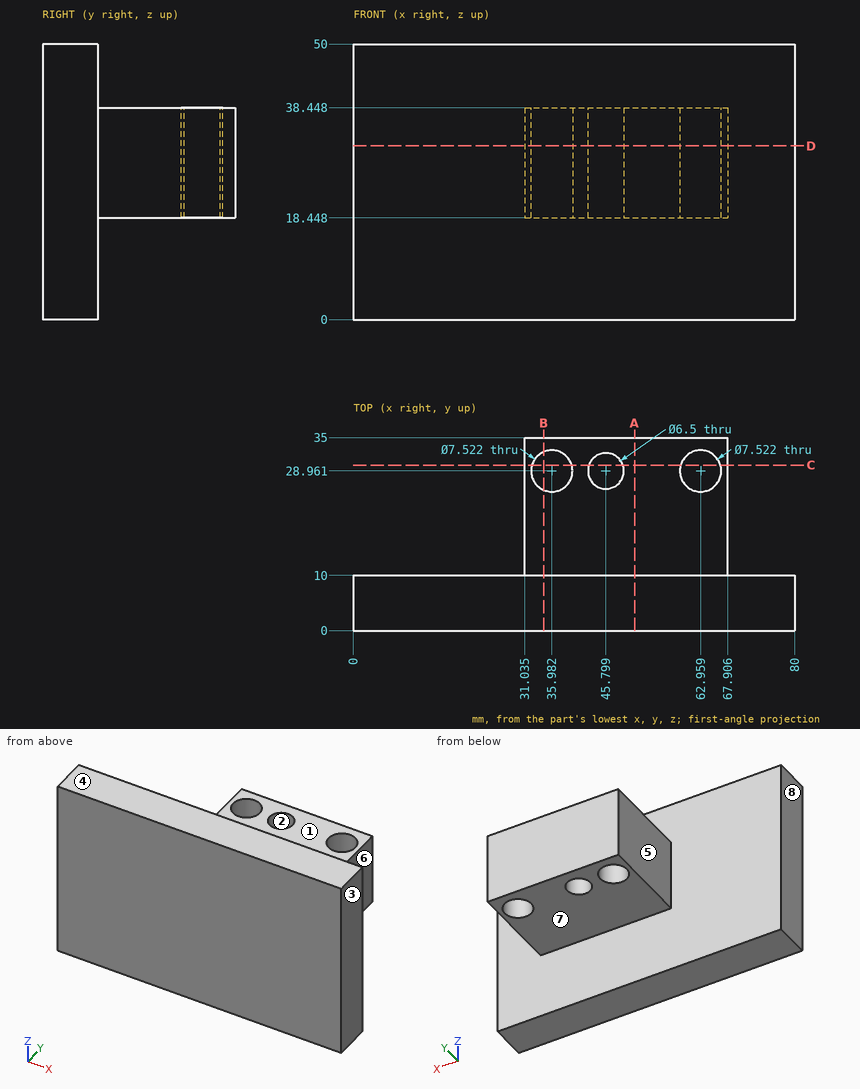
Can you work these out from the drawing? Everything is in mm from the part's minimum corner. A direction names the side the tool comes from. Coordinates: 2 decimals unless noted, no trailing zeros. Loops run counter-clockwise (first coordinate to the right, second up) from the corner with the lowest first, then second, coordinate; pieces in that order, holes last. Notation, with made-up numbers: (-19.75, 34.25) - (-12.75, 34.25) arc R19 cw to (-12.75, 57.25) - close; hole circle Ø6 at (-36, -20). An arc over 180 degrees is marked (long way). Put each result on its own line as item: value. Start each with the question number.
Item 1: For pin 1 (16 mm diameter, centred on y = 25.5, z = 26.5, fed in from -X) (1 decimal); pin 2 (20 mm diameter, centred on x = 49.5, y = 25.5, fed in from +Z); pin 3 (10 mm diameter, centred on x = 62.5, z = 8.5, fed in from +Y), each with a flat end and sliding along its axis, tell me the tip position at first contact or that it passes through.
Item 2: If we mould it in two halves opening along X, with no side actions, what happens to the marked faces 1, 2 and 3? For each: +X half, -X half, draft (parallel to the pull), parting line (faces both ways), or undercut.
Item 3: Suppose I cut it at C-C (y = 30). Please give me the cut outline in (x, z) (1 decimal), and give its area (3 significant figures).
Item 4: Suppose I cut it at D-D (z = 31.5). State how many separate pieces and enclosed holes the cut face has, and give its area (3 significant figures).
Item 5: If I drill on line 1 along Y through (x, z) = (56.5, 4); line 2 along X through (y, z) = (33.5, 22) (1 decimal), over which ranges is the centre line in solid material (lowest first)?
Item 6: Which directions (+Z, -Z, +X, -X, +Y, -Y) give clear straight access to the entire face, cutting with the end or side of a thin tool? Please do the marked faces 4, 5, 6, 7 and 8.
Item 7: Suppose I cut it at A-A (x = 51). Please give me the cut outline in (y, z), and give its area (3 significant figures).
Item 8: Suppose I cut it at B-B (x = 34.5). Please give me the cut outline in (y, z) (1 decimal), and give its area (3 significant figures).
Here are the results:
1. pin 1: x = 31
1. pin 2: z = 38.45
1. pin 3: y = 10
2. face 1: draft
2. face 2: undercut
2. face 3: +X half
3. outline: (31, 18.4) - (32.4, 18.4) - (32.4, 38.4) - (31, 38.4) - close; (39.6, 18.4) - (42.7, 18.4) - (42.7, 38.4) - (39.6, 38.4) - close; (48.9, 18.4) - (59.3, 18.4) - (59.3, 38.4) - (48.9, 38.4) - close; (66.6, 18.4) - (67.9, 18.4) - (67.9, 38.4) - (66.6, 38.4) - close
3. area: 325 mm²
4. separate pieces: 1
4. enclosed holes: 3
4. area: 1,600 mm²
5. line 1: 0 to 10
5. line 2: 31 to 67.9
6. face 4: +Z, +X, -X, +Y, -Y
6. face 5: +Z, -Z, -X, +Y
6. face 6: +Z, -Z, +X, +Y
6. face 7: -Z, +X, -X, +Y
6. face 8: +Z, -Z, -X, +Y, -Y
7. outline: (0, 0) - (10, 0) - (10, 18.45) - (35, 18.45) - (35, 38.45) - (10, 38.45) - (10, 50) - (0, 50) - close
7. area: 1,000 mm²
8. outline: (0, 0) - (10, 0) - (10, 18.4) - (25.5, 18.4) - (25.5, 38.4) - (10, 38.4) - (10, 50) - (0, 50) - close; (32.4, 18.4) - (35, 18.4) - (35, 38.4) - (32.4, 38.4) - close
8. area: 862 mm²
